from build123d import *

# Parameters (mm, degrees)
CROQUIS1_W              = 36
CROQUIS1_H              = 35
SALIENTE_EXTRUIR1_DEPTH = 20
CROQUIS2_W              = 36
CROQUIS2_H              = 33
CORTAR_EXTRUIR1_DEPTH   = 7
CROQUIS3_W              = 32
CROQUIS3_H              = 31
CORTAR_EXTRUIR2_DEPTH   = 11
CORTAR_EXTRUIR3_REACH   = 46.147
CROQUIS4_W              = 8.7
CROQUIS4_H              = 4
CORTAR_EXTRUIR4_REACH   = 46.147
CROQUIS5_W              = 10
CROQUIS5_H              = 1
CROQUIS6_W              = 10
CROQUIS6_H              = 1
CORTAR_EXTRUIR5_DEPTH   = 1
CORTAR_EXTRUIR6_DEPTH   = 1
CORTAR_EXTRUIR7_DEPTH   = 1.2


with BuildPart() as part:
    # Croquis1 → Saliente-Extruir1 (new body)
    with BuildSketch(Plane(origin=(0, 0, 0), x_dir=(1, 0, 0), z_dir=(0, 1, 0))):
        Rectangle(CROQUIS1_W, CROQUIS1_H)
    extrude(amount=SALIENTE_EXTRUIR1_DEPTH)

    # Croquis2 → Cortar-Extruir1 (cut)
    with BuildSketch(Plane(origin=(0, 20, 0), x_dir=(1, 0, 0), z_dir=(0, 1, 0))):
        with Locations((0, 1)):
            Rectangle(CROQUIS2_W, CROQUIS2_H)
    extrude(amount=-CORTAR_EXTRUIR1_DEPTH, mode=Mode.SUBTRACT)

    # Croquis3 → Cortar-Extruir2 (cut)
    with BuildSketch(Plane(origin=(0, 13, 0), x_dir=(1, 0, 0), z_dir=(0, 1, 0))):
        Rectangle(CROQUIS3_W, CROQUIS3_H)
    extrude(amount=-CORTAR_EXTRUIR2_DEPTH, mode=Mode.SUBTRACT)

    # Croquis4 → Cortar-Extruir3 (cut, up to next)
    with BuildSketch(Plane.XY.offset(17.5), mode=Mode.PRIVATE) as cortar_extruir3_sk1:
        with Locations((-7.65, 6)):
            Rectangle(CROQUIS4_W, CROQUIS4_H)
    cortar_extruir3_tool1 = extrude(cortar_extruir3_sk1.sketch, amount=-CORTAR_EXTRUIR3_REACH, mode=Mode.PRIVATE) & part.part
    add(cortar_extruir3_tool1.solids().sort_by_distance((-7.65, 6, 17.5))[0], mode=Mode.SUBTRACT)

    # Croquis5 → Cortar-Extruir4 (cut, up to next)
    with BuildSketch(Plane.XY.offset(17.5), mode=Mode.PRIVATE) as cortar_extruir4_sk1:
        with Locations((0, 17)):
            Rectangle(CROQUIS5_W, CROQUIS5_H)
    cortar_extruir4_tool1 = extrude(cortar_extruir4_sk1.sketch, amount=-CORTAR_EXTRUIR4_REACH, mode=Mode.PRIVATE) & part.part
    add(cortar_extruir4_tool1.solids().sort_by_distance((0, 17, 17.5))[0], mode=Mode.SUBTRACT)

    # Croquis6 → Cortar-Extruir5 (cut)
    with BuildSketch(Plane.XY.offset(17.5)):
        with Locations((0, 18)):
            Rectangle(CROQUIS6_W, CROQUIS6_H)
    extrude(amount=-CORTAR_EXTRUIR5_DEPTH, mode=Mode.SUBTRACT)

    # Croquis7 → Cortar-Extruir6 (cut)
    with BuildSketch(Plane(origin=(0, 13, 0), x_dir=(1, 0, 0), z_dir=(0, 1, 0))):
        Polygon((-18, -15.5), (-17, -15.5), (-17, 16.3), (17, 16.3), (17, -15.5), (18, -15.5), (18, 17.5), (-18, 17.5), align=None)
    extrude(amount=-CORTAR_EXTRUIR6_DEPTH, mode=Mode.SUBTRACT)

    # Croquis8 → Cortar-Extruir7 (cut)
    with BuildSketch(Plane(origin=(0, 0, -17.5), x_dir=(-1, 0, 0), z_dir=(0, 0, -1))):
        Polygon((-5, 12), (-5, 7), (5, 7), (5, 12), (3.5, 12), (3.5, 9), (-3.5, 9), (-3.5, 12), align=None)
    extrude(amount=-CORTAR_EXTRUIR7_DEPTH, mode=Mode.SUBTRACT)


solid = part.part
CAD build for the part. Positions are in the model's coordinates, mm. A direction names the side the tool comes from. Coordinates: 2 decimals unless noted, no trailing zeros. Loops run counter-clockwise (first coordinate to the right, second up) from the corner with the lowest first, then second, coordinate; pieces in that order, holes last. Notation, with made-up numbers: (-36.75, -26.75) -> (-21.75, -26.75) arc R10 cw to (-21.75, -10.75) -> close; hole circle Ø7 at (-23.5, 3.5). An arc over 180 degrees is marked (long way). One line per item, written item: value.
1. Drill centre lines: line 1 (Z direction, x = 14, y = 2.5); line 2 (X direction, y = 2.5, z = -12.5); line 3 (Y direction, x = 15.5, z = 14). Where is each one in solid material? Low to high. Write a range as [from, to].
Answers:
line 1: z = [-17.5, -15.5], [15.5, 17.5]
line 2: x = [-18, -16], [16, 18]
line 3: y = [0, 2]
2. Flat gauge pins, fed straight in: P1, Ø2, axis at x = -8, z = 17, coming from the -Y side; P2, Ø0.8, axis at x = -2, y = 18, coming from the +Z side; P3, Ø0.8, axis at y = 12.5, z = 2.5, coming from the -X side. Where does each tip first touch, or does it go through?
Answers:
P1: stops at y = 0
P2: stops at z = 16.5
P3: stops at x = -17
3. Slice it at A-A on x = -11. Write the cut outline in (y, z).
Answers:
outline: (0, -17.5) -> (12, -17.5) -> (12, -16.3) -> (13, -16.3) -> (13, -15.5) -> (2, -15.5) -> (2, 15.5) -> (4, 15.5) -> (4, 17.5) -> (0, 17.5) -> close; (8, 15.5) -> (20, 15.5) -> (20, 17.5) -> (8, 17.5) -> close
4. Pull direction X, two halves, no side cores. Call faces 6 (the face through (0, 12, -17)), 7 (the face through (-17, 12.5, -0.2)), 8 (the face through (0, 9, -17)): pulls with the +X half, pulls with the -X half, needs draft (parallel to the pull), parting line crosses it, or undercut.
Answers:
face 6: needs draft
face 7: pulls with the -X half
face 8: undercut
5. Slice it at D-D on x = 13.5. Write the cut outline in (y, z), and give its area (3 significant figures).
Answers:
outline: (0, -17.5) -> (12, -17.5) -> (12, -16.3) -> (13, -16.3) -> (13, -15.5) -> (2, -15.5) -> (2, 15.5) -> (20, 15.5) -> (20, 17.5) -> (0, 17.5) -> close
area: 127 mm^2
6. Which spindle directions (+Z, -Z, +X, -X, +Y, -Y) get a long thin tool onto all of the face, cutting with end or side? Do faces 1 (the face through (0, 11, 15.5)), 2 (the face through (5, 10, -17)), 3 (the face through (-8, 4, 17)), 4 (the face through (17, 12.5, -0.6)), 5 (the face through (0, 17.5, 16)). Say none if no direction does.
Answers:
face 1: +Y
face 2: -Z, +Y
face 3: +Z
face 4: -Z, +X, +Y
face 5: +Z, -Z
7. Slice it at B-B on y = 11.5. Write the cut outline in (x, z), and give its area (3 significant figures).
Answers:
outline: (-18, -17.5) -> (-5, -17.5) -> (-5, -16.3) -> (-3.5, -16.3) -> (-3.5, -17.5) -> (3.5, -17.5) -> (3.5, -16.3) -> (5, -16.3) -> (5, -17.5) -> (18, -17.5) -> (18, 17.5) -> (-18, 17.5) -> close; hole (-16, -15.5) -> (16, -15.5) -> (16, 15.5) -> (-16, 15.5) -> close
area: 264 mm^2
8. Slice it at C-C on z = 5. Write the cut outline in (x, y).
Answers:
outline: (-18, 0) -> (18, 0) -> (18, 12) -> (17, 12) -> (17, 13) -> (16, 13) -> (16, 2) -> (-16, 2) -> (-16, 13) -> (-17, 13) -> (-17, 12) -> (-18, 12) -> close
